Autodesk Inventor part; units mm, degrees
ref_plane "YZ Plane" through (0, 0, 0) normal (1, 0, 0) x (0, 1, 0)
ref_plane "XZ Plane" through (0, 0, 0) normal (0, 1, 0) x (-1, 0, 0)
ref_plane "XY Plane" through (0, 0, 0) normal (0, 0, 1) x (1, 0, 0)
sketch "Sketch1" plane through (0, 0, 0) normal (0, 0, 1) x (1, 0, 0)
  line L0 (-8.5, -5) -> (8.5, -5)
  line L1 (8.5, -5) -> (8.5, 5)
  line L2 (8.5, 5) -> (-8.5, 5)
  line L3 (-8.5, 5) -> (-8.5, -5)
  line L4 (-8.5, -5) -> (8.5, 5) construction
  line L5 (8.5, -5) -> (-8.5, 5) construction
  line L6 (0, -7) -> (0, 7) construction
  line L7 (-7, -3.4) -> (7, -3.4)
  line L8 (7, -3.4) -> (7, 1.6)
  line L9 (7, 1.6) -> (-7, 1.6)
  line L10 (-7, 1.6) -> (-7, -3.4)
  line L11 (-7, -3.4) -> (7, 1.6) construction
  line L12 (7, -3.4) -> (-7, 1.6) construction
  point P0 (0, 0)
  point P1 (0, -0.9)
  dimension "d0" = 10
  dimension "d1" = 17
  dimension "d2" = 4.1
  dimension "d3" = 5
  dimension "d4" = 14
extrude "Extrusion1" add sketch "Sketch1" along normal blind 1
fillet "Fillet1" radius 1 4 edges at (8.5, 5, 0.5) (8.5, -5, 0.5) (-8.5, -5, 0.5) (-8.5, 5, 0.5)
fillet "Fillet2" radius 1 4 edges at (7, 1.6, 0.5) (7, -3.4, 0.5) (-7, -3.4, 0.5) (-7, 1.6, 0.5)
properties part number "CAMERA_CON_SPACER"
Verification items for the finished model (mm, model axes). A direction names the side the tool comes from. Give positions to 0.01 mm unless a question says otherwise; leave off trailing zeros. Loops run counter-clockwise (first coordinate to the right, second up) from the corner with the lowest first, then second, coordinate; pieces in that order, holes last.
1. Cross-section at C-C on x = -5.75. Record the cut outline in (y, z).
Derived:
outline: (-5, 0) - (-3.4, 0) - (-3.4, 1) - (-5, 1) - close; (1.6, 0) - (5, 0) - (5, 1) - (1.6, 1) - close
2. Release check for a two-part mould opening along X. For faces 3 (the cylindrical face through (6.715, 1.299, 0.507)), 4 (the cylindrical face through (-8.199, 4.715, 0.507)), 5 (the flat face through (8.5, -0.1, 0.5)) record: +X half, -X half, draft (parallel to the pull), parting line (faces both ways), or undercut.
Derived:
face 3: undercut
face 4: -X half
face 5: +X half
3. Go/stop test with a flat-tipped pin: P1, Ø1.5, axis at x = -3, y = -2, coming from the +Z side. Record where the tip stops, or that it passes through.
Derived:
P1: passes through
4. Cross-section at B-B on z = 0.75. Record the cut outline in (x, y), and give its area (3 significant figures).
Derived:
outline: (-8.5, -4) arc R1 ccw to (-7.5, -5) - (7.5, -5) arc R1 ccw to (8.5, -4) - (8.5, 4) arc R1 ccw to (7.5, 5) - (-7.5, 5) arc R1 ccw to (-8.5, 4) - close; hole (-7, -2.4) arc R1 ccw to (-6, -3.4) - (6, -3.4) arc R1 ccw to (7, -2.4) - (7, 0.6) arc R1 ccw to (6, 1.6) - (-6, 1.6) arc R1 ccw to (-7, 0.6) - close
area: 100 mm2
5. Cross-section at A-A on y = -0.75. Record the cut outline in (x, z).
Derived:
outline: (-8.5, 0) - (-7, 0) - (-7, 1) - (-8.5, 1) - close; (7, 0) - (8.5, 0) - (8.5, 1) - (7, 1) - close
6. Tool access check on faces 1 (the cylindrical face through (8.215, 4.699, 0.507)), 2 (the cylindrical face through (-6.699, 1.315, 0.507)). Record the directions out of +Z, -Z, +X, -X, +Y, -Y that give a thin tool (end or side, any length) a straight path to the whole face; none if there is none.
Derived:
face 1: +Z, -Z, +X, +Y
face 2: +Z, -Z
7. Material ranges on probe 1 along Y at (x, z) = (0.75, 0.6); probe 2 along X at (y, z) = (0.5, 0.2); probe 3 along X at (y, z) = (-3, 0.1), recorded low to high.
Derived:
probe 1: y = -5 to -3.4, 1.6 to 5
probe 2: x = -8.5 to -7, 7 to 8.5
probe 3: x = -8.5 to -6.8, 6.8 to 8.5
